```python
from build123d import *

# Parameters (mm, degrees)
SKIZZE1_W                       = 17.5
SKIZZE1_H                       = 18.5
AUFSATZ_LINEAR_AUSTRAGEN1_DEPTH = 1.5
VERRUNDUNG1_R                   = 0.5
SCHNITT_LINEAR_AUSTRAGEN1_REACH = 21.851
VERRUNDUNG2_R                   = 0.5
SCHL_SSELLOCH_DEPTH             = 1.5
SKIZZE6_W                       = 3.103008178
SKIZZE6_H                       = 0.25
GRIFF_DEPTH                     = 1.5
LANGLOCH_ANTENNE_START          = -1.5
LANGLOCH_ANTENNE_DEPTH          = 1.5
SCHNITT_LINEAR_AUSTRAGEN2_DEPTH = 1.5


with BuildPart() as part:
    # Skizze1 → Aufsatz-Linear austragen1 (new body)
    with BuildSketch(Plane(origin=(0, 0, 0), x_dir=(1, 0, 0), z_dir=(0, 1, 0))):
        Rectangle(SKIZZE1_W, SKIZZE1_H)
    extrude(amount=AUFSATZ_LINEAR_AUSTRAGEN1_DEPTH)

    # Verrundung1
    verrundung1_edges = [part.edges().sort_by_distance(p)[0] for p in [
        (-8.75, 1.5, 0),
        (8.75, 1.5, 0),
        (0, 1.5, -9.25),
    ]]
    fillet(verrundung1_edges, radius=VERRUNDUNG1_R)

    # Schnitt-Linear austragen1: up to this face of the body (flat: up to its plane)
    schnitt_linear_austragen1_end = Plane(part.part.faces().sort_by_distance((8.75, 0.5, 0))[0])
    # Skizze2 → Schnitt-Linear austragen1 (cut, up to the picked face)
    with BuildSketch(Plane.ZY.offset(8.75), mode=Mode.PRIVATE) as schnitt_linear_austragen1_sk1:
        Polygon((9.25, 0), (8.5, 1.5), (9.25, 1.5), align=None)
    schnitt_linear_austragen1_tool1 = split(extrude(schnitt_linear_austragen1_sk1.sketch, amount=-SCHNITT_LINEAR_AUSTRAGEN1_REACH, mode=Mode.PRIVATE), bisect_by=schnitt_linear_austragen1_end, keep=Keep.BOTH, mode=Mode.PRIVATE)
    add(schnitt_linear_austragen1_tool1.solids().sort_by(Axis((-8.75, 1, 9), (1, 0, 0)))[0], mode=Mode.SUBTRACT)

    # Verrundung2
    # the kernel refuses this fillet: 0.5 mm, written as the material it takes off along each edge
    with BuildSketch(Plane(origin=(-8.25, 1, -8.75), x_dir=(-1, 0, 0), z_dir=(0, 0, -1))) as verrundung2_piece_1_section:
        Polygon((0, 0), (VERRUNDUNG2_R, 0), (VERRUNDUNG2_R, VERRUNDUNG2_R), (0, VERRUNDUNG2_R), align=None)
    verrundung2_piece_1 = extrude(amount=VERRUNDUNG2_R, mode=Mode.PRIVATE)
    verrundung2_piece_1 = verrundung2_piece_1 - Plane(origin=(-8.25, 1, -8.75), x_dir=(0.7071067811865475, -0.7071067811865475, 0), z_dir=(0, 0, -1)) * Sphere(VERRUNDUNG2_R, mode=Mode.PRIVATE)
    add(verrundung2_piece_1, mode=Mode.SUBTRACT)
    with BuildSketch(Plane(origin=(8.25, 1, -8.75), x_dir=(0, 0, -1), z_dir=(1, 0, 0))) as verrundung2_piece_2_section:
        Polygon((0, 0), (VERRUNDUNG2_R, 0), (VERRUNDUNG2_R, VERRUNDUNG2_R), (0, VERRUNDUNG2_R), align=None)
    verrundung2_piece_2 = extrude(amount=VERRUNDUNG2_R, mode=Mode.PRIVATE)
    verrundung2_piece_2 = verrundung2_piece_2 - Plane(origin=(8.25, 1, -8.75), x_dir=(0, -0.7071067811865475, 0.7071067811865475), z_dir=(1, 0, 0)) * Sphere(VERRUNDUNG2_R, mode=Mode.PRIVATE)
    add(verrundung2_piece_2, mode=Mode.SUBTRACT)
    with BuildSketch(Plane(origin=(8.75, -1.25, -9.25), x_dir=(0, 0, 1), z_dir=(0, 1, 0)), Plane(origin=(-8.75, -1.25, -9.25), x_dir=(1, 0, 0), z_dir=(0, 1, 0))) as verrundung2_piece_3:
        with BuildLine():
            CenterArc((VERRUNDUNG2_R, -VERRUNDUNG2_R), VERRUNDUNG2_R, 90, 90)
            Line((0, -VERRUNDUNG2_R), (0, 0))
            Line((0, 0), (VERRUNDUNG2_R, 0))
        make_face()
    extrude(amount=2.25, mode=Mode.SUBTRACT)

    # Skizze5 → Schlüsselloch (cut)
    with BuildSketch(Plane(origin=(0, 1.5, 0), x_dir=(1, 0, 0), z_dir=(0, 1, 0))):
        with BuildLine():
            Line((-3.5, 6.35), (-3.5, 4.35))
            Line((-3.5, 4.35), (-1.732050808, 4.35))
            ThreePointArc((-1.732050808, 4.35), (-2, 5.35), (-1.732050808, 6.35))
            Line((-1.732050808, 6.35), (-3.5, 6.35))
        make_face()
        with BuildLine():
            ThreePointArc((1.732050808, 6.35), (0, 7.35), (-1.732050808, 6.35))
            Line((-1.732050808, 6.35), (1.732050808, 6.35))
        make_face()
        with BuildLine():
            ThreePointArc((-1.732050808, 6.35), (-2, 5.35), (-1.732050808, 4.35))
            Line((-1.732050808, 4.35), (1.732050808, 4.35))
            ThreePointArc((1.732050808, 4.35), (1.931851653, 4.83236191), (2, 5.35))
            ThreePointArc((2, 5.35), (1.931851653, 5.86763809), (1.732050808, 6.35))
            Line((1.732050808, 6.35), (-1.732050808, 6.35))
        make_face()
        with BuildLine():
            Line((1.732050808, 4.35), (-1.732050808, 4.35))
            ThreePointArc((-1.732050808, 4.35), (0, 3.35), (1.732050808, 4.35))
        make_face()
        with BuildLine():
            ThreePointArc((2, 5.35), (1.931851653, 4.83236191), (1.732050808, 4.35))
            Line((1.732050808, 4.35), (3.5, 4.35))
            Line((3.5, 4.35), (3.5, 6.35))
            Line((3.5, 6.35), (1.732050808, 6.35))
            ThreePointArc((1.732050808, 6.35), (1.931851653, 5.86763809), (2, 5.35))
        make_face()
    extrude(amount=-SCHL_SSELLOCH_DEPTH, mode=Mode.SUBTRACT)

    # Skizze6 → Griff (cut)
    with BuildSketch(Plane(origin=(0, 1.5, 0), x_dir=(1, 0, 0), z_dir=(0, 1, 0))):
        with Locations((0, -8.875)):
            Rectangle(SKIZZE6_W, SKIZZE6_H)
    extrude(amount=-GRIFF_DEPTH, mode=Mode.SUBTRACT)

    # Skizze7 → Langloch_Antenne (cut)
    with BuildSketch(Plane(origin=(0, 1.5, 0), x_dir=(1, 0, 0), z_dir=(0, 1, 0)).offset(LANGLOCH_ANTENNE_START)):
        with BuildLine():
            Line((0.75, 9.25), (0.75, -4.75))
            ThreePointArc((0.75, -4.75), (0, -5.5), (-0.75, -4.75))
            Line((-0.75, -4.75), (-0.75, 9.25))
            ThreePointArc((-0.75, 9.25), (0, 10), (0.75, 9.25))
        make_face()
    extrude(amount=LANGLOCH_ANTENNE_DEPTH, mode=Mode.SUBTRACT)

    # Skizze8 → Schnitt-Linear austragen2 (cut)
    with BuildSketch(Plane(origin=(0, 1.5, 0), x_dir=(1, 0, 0), z_dir=(0, 1, 0))):
        Polygon((3.5, 4.35), (0.75, 3.495950378), (-0.75, 3.495950378), (-3.5, 4.35), (-3.5, 6.35), (-0.75, 7.204049622), (0.75, 7.204049622), (3.5, 6.35), align=None)
    extrude(amount=-SCHNITT_LINEAR_AUSTRAGEN2_DEPTH, mode=Mode.SUBTRACT)


solid = part.part
```
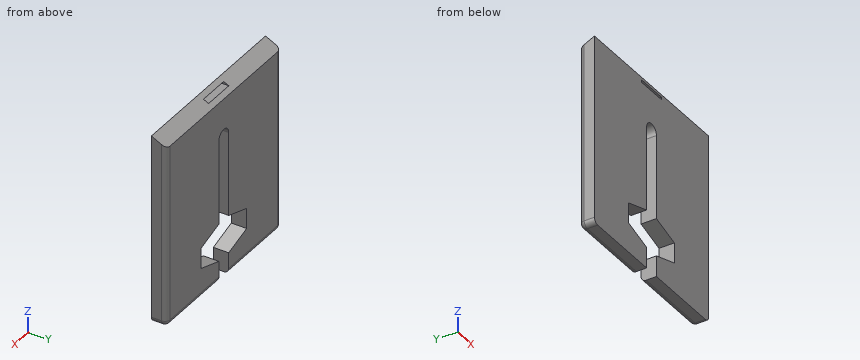
Can you work these out from the model? Positions are in its coordinate system, mm. Round coordinates to 2 decimals unless told otherwise and drop trailing zeros. Loops run counter-clockwise (first coordinate to the right, second up) from the corner with the lowest first, then second, coordinate; pieces in that order, holes last. Notation, with made-up numbers: M 10.25,32 L 60.25,32 A34 cw 60.25,67 Z; hole C 0,53 d2. An arc over 180 degrees is marked long. Answer as a JSON object with one key per item and string values. Group by question number.
Q1. Imagine slicing it at B-B, the plane x = 0. Please give me the cut outline in (y, z).
Q2. Imagine slicing it at A-A, the plane z = 1. Please give me the cut outline in (x, y), then the cut area to 3 significant figures.
Q3. Please list where these lines run through material, in increasing order: L1, parallel to X at y = 0.8, z = -7.75; L2, parallel to X at y = 0.5, z = -6; L3, parallel to Z at x = 4.25, y = 1.
Q4. Will this pin go through, and if not, where does the flat tip stop? pin 1 (0.5 mm diameter, centred on x = 0.5, y = 0.5, fed in from +Z) (3 decimals).
Q5. Imagine slicing it at D-D, the plane z = -4.75. Please give me the cut outline in (x, y), then the cut area to 3 significant figures.
Q6. Imagine slicing it at C-C, the plane x = -7.25. Please give me the cut outline in (y, z), then the cut area to 3 significant figures.
Findings:
{
 "1": {"outline": "M 0,5.5 L 1.5,5.5 L 1.5,8.5 L 1,8.75 L 0,8.75 Z; M 0,9 L 0.5,9 L 0,9.25 Z"},
 "2": {"outline": "M -8.75,0 L -0.75,0 L -0.75,1.5 L -8.25,1.5 A0.5 ccw -8.75,1 Z; M 0.75,0 L 8.75,0 L 8.75,1 A0.5 ccw 8.25,1.5 L 0.75,1.5 Z", "area": "23.9 mm2"},
 "3": {"L1": "x = -8.75 to -0.75, 0.75 to 8.75", "L2": "x = -8.75 to -3.5, 3.5 to 8.75", "L3": "z = -9.25 to 8.75"},
 "4": {"pin 1": "stops at z = 9.125"},
 "5": {"outline": "M -8.75,0 L -3.5,0 L -3.5,1.5 L -8.25,1.5 A0.5 ccw -8.75,1 Z; M 3.5,0 L 8.75,0 L 8.75,1 A0.5 ccw 8.25,1.5 L 3.5,1.5 Z", "area": "15.6 mm2"},
 "6": {"outline": "M 0,-9.25 L 1,-9.25 A0.5 ccw 1.5,-8.75 L 1.5,8.5 L 0,9.25 Z", "area": "27.1 mm2"}
}
